```python
from build123d import *

# Parameters (mm, degrees)
EXTRUDE008_DEPTH = 1.5
CIRCLE_R         = 2.5
EXTRUDE007_DEPTH = 20


with BuildPart() as extrude008:
    # Polygon → Extrude008 (new body)
    with BuildSketch(Plane.XY):
        with BuildLine():
            Line((2.453739, 3.75), (4.474465, 0.25))
            ThreePointArc((4.474465, 0.25), (4.541452, 0), (4.474465, -0.25))
            Line((4.474465, -0.25), (2.453739, -3.75))
            ThreePointArc((2.453739, -3.75), (2.270726, -3.933013), (2.020726, -4))
            Line((2.020726, -4), (-2.020726, -4))
            ThreePointArc((-2.020726, -4), (-2.270726, -3.933013), (-2.453739, -3.75))
            Line((-2.453739, -3.75), (-4.474465, -0.25))
            ThreePointArc((-4.474465, -0.25), (-4.541452, 0), (-4.474465, 0.25))
            Line((-4.474465, 0.25), (-2.453739, 3.75))
            ThreePointArc((-2.453739, 3.75), (-2.270726, 3.933013), (-2.020726, 4))
            Line((-2.020726, 4), (2.020726, 4))
            ThreePointArc((2.020726, 4), (2.270726, 3.933013), (2.453739, 3.75))
        make_face()
    extrude(amount=EXTRUDE008_DEPTH)


with BuildPart() as vis:
    # Circle → Extrude007 (new body)
    with BuildSketch(Plane(origin=(0, 0, 0), x_dir=(1, 0, 0), z_dir=(0, 0, -1))):
        Circle(CIRCLE_R)
    extrude(amount=-EXTRUDE007_DEPTH)

    # Fusion004: union Extrude008
    add(extrude008.part)


with BuildPart() as vis_1:
    # Fusion004 placement: moved
    add(vis.part.moved(Location((25, 50, -5))))


solid = vis_1.part
```
Part model, mm, in its own coordinate system. A direction names the side the tool comes from. Give positions to 0.01 mm unless a question says otherwise; leave off trailing zeros. Write each loop counter-clockwise with the first axis right and the second up, starting at its lowest first coordinate (ties: lowest second). Pieces come first, ordered by that corner, then holes. Notation, with made-up numbers: (55, -25) -> (66, -25) arc R6 cw to (66, -17) -> close; hole circle Ø11 at (66, 67.5). An arc over 180 degrees is marked (long way). Put each result on its own line as item: value. Start each with the question number.
Item 1: Cut at B-B (x = 25). List the corners of the cut face in (y, z).
Item 2: Cut at A-A (y = 50). List the corners of the cut face in (x, z).
Item 3: Cut at C-C (z = 12). List the corners of the cut face in (x, y), then the cut area to 3 significant figures.
Item 4: Wall check: L1, parallel to Z at x = 22.5, y = 49.5; L2, parallel to X at y = 49.5, z = -3; L3, parallel to X at y = 50, z = 4. Give the ranges that are in metal, low to high. Write a range as [from, to].
Item 5: Pin check, flat tips, straight feed: pin 1 Ø1 at (y, z) = (50.5, 3.5) entering from -X; pin 2 Ø1.5 at (x, y) = (28.5, 47) entering from +Z; pin 3 Ø3 at (y, z) = (53, 6) entering from +X. Stop position of each tip, or through.
Item 6: Cut at D-D (x = 21.5). List the corners of the cut face in (y, z), then the cut area to 3 significant figures.
Item 7: Which spindle directions (+Z, -Z, +X, -X, +Y, -Y) get a long thin tool onto all of the face, cutting with end or side? Do faces 1 (the face through (25, 50, -5)), 2 (the face through (23, 48, -3.5)). Say none if no direction does.
Answer list:
1. outline: (46, -5) -> (54, -5) -> (54, -3.5) -> (52.5, -3.5) -> (52.5, 15) -> (47.5, 15) -> (47.5, -3.5) -> (46, -3.5) -> close
2. outline: (20.46, -5) -> (29.54, -5) -> (29.54, -3.5) -> (27.5, -3.5) -> (27.5, 15) -> (22.5, 15) -> (22.5, -3.5) -> (20.46, -3.5) -> close
3. outline: circle Ø5 at (25, 50)
3. area: 19.6 mm2
4. L1: z = [-5, -3.5]
4. L2: x = [22.55, 27.45]
4. L3: x = [22.5, 27.5]
5. pin 1: stops at x = 22.5
5. pin 2: stops at z = -3.5
5. pin 3: stops at x = 27
6. outline: (48.06, -5) -> (51.94, -5) -> (51.94, -3.5) -> (48.06, -3.5) -> close
6. area: 5.81 mm2
7. face 1: -Z, +X, -X, +Y, -Y
7. face 2: +Z
